from build123d import *

# Parameters (mm, degrees)
BOSS_EXTRU_2_DEPTH       = 73
ESQUISSE7_R              = 1.75
ENL_V_MAT_EXTRU_4_DEPTH  = 12
ENL_V_START              = -5.6
ENL_V_MAT_EXTRU_5_DEPTH  = 2.6
ENL_V_START_2            = -12
ESQUISSE12_R             = 1.75
ENL_V_MAT_EXTRU_6_DEPTH  = 12
ENL_V_START_3            = -3
ENL_V_MAT_EXTRU_7_DEPTH  = 2.6
ESQUISSE21_W             = 15
ESQUISSE21_H             = 17
ENL_V_MAT_EXTRU_14_DEPTH = 79.208055851
ESQUISSE22_W             = 2
ESQUISSE22_H             = 6
ENL_V_MAT_EXTRU_15_DEPTH = 79.208055851
ENL_V_START_4            = -17
ENL_V_MAT_EXTRU_17_DEPTH = 6
ENL_V_START_5            = -23
ENL_V_MAT_EXTRU_19_DEPTH = 6
CHANFREIN1_SIZE          = 4
CHANFREIN2_SIZE          = 4


with BuildPart() as part:
    # Esquisse3 → Boss.-Extru.2 (new body)
    with BuildSketch(Plane.XY):
        with BuildLine():
            ThreePointArc((-26.024027359, 27), (0, 37.5), (26.024027359, 27))
            Line((26.024027359, 27), (13.076696831, 27))
            Line((13.076696831, 27), (-13.076696831, 27))
            Line((-13.076696831, 27), (-26.024027359, 27))
        make_face()
    extrude(amount=BOSS_EXTRU_2_DEPTH)

    # Esquisse7 → Enlèv. mat.-Extru.4 (cut)
    with BuildSketch(Plane.XY.offset(73)):
        with Locations((-12.915565842, 31.180934222)):
            Circle(ESQUISSE7_R)
        with Locations((12.915565842, 31.180934222)):
            Circle(ESQUISSE7_R)
    extrude(amount=-ENL_V_MAT_EXTRU_4_DEPTH, mode=Mode.SUBTRACT)

    # Esquisse11 → Enlèv. mat.-Extru.5 (cut)
    with BuildSketch(Plane.XY.offset(73).offset(ENL_V_START)):
        with BuildLine():
            Line((-15.765565842, 31.180934222), (-15.765565842, 34.024945756))
            ThreePointArc((-15.765565842, 34.024945756), (-12.95813326, 35.190009696), (-10.065565842, 36.123875543))
            Line((-10.065565842, 36.123875543), (-10.065565842, 29.426382489))
            Line((-10.065565842, 29.426382489), (-12.915565842, 27.780934222))
            Line((-12.915565842, 27.780934222), (-15.765565842, 29.426382489))
            Line((-15.765565842, 29.426382489), (-15.765565842, 31.180934222))
        make_face()
        with BuildLine():
            Line((10.065565842, 36.123875543), (10.065565842, 29.426382489))
            Line((10.065565842, 29.426382489), (12.915565842, 27.780934222))
            Line((12.915565842, 27.780934222), (15.765565842, 29.426382489))
            Line((15.765565842, 29.426382489), (15.765565842, 34.024945756))
            ThreePointArc((15.765565842, 34.024945756), (12.95813326, 35.190009696), (10.065565842, 36.123875543))
        make_face()
    extrude(amount=ENL_V_MAT_EXTRU_5_DEPTH, mode=Mode.SUBTRACT)

    # Esquisse12 → Enlèv. mat.-Extru.6 (cut)
    with BuildSketch(Plane(origin=(0, 0, 0), x_dir=(-1, 0, 0), z_dir=(0, 0, -1)).offset(ENL_V_START_2)):
        with Locations(Location((-12.915565842, 31.180934222, 0), (0, 0, 180))):
            Circle(ESQUISSE12_R)
        with Locations(Location((12.915565842, 31.180934222, 0), (0, 0, 180))):
            Circle(ESQUISSE12_R)
    extrude(amount=ENL_V_MAT_EXTRU_6_DEPTH, mode=Mode.SUBTRACT)

    # Esquisse14 → Enlèv. mat.-Extru.7 (cut)
    with BuildSketch(Plane(origin=(0, 0, 0), x_dir=(-1, 0, 0), z_dir=(0, 0, -1)).offset(ENL_V_START_3)):
        with BuildLine():
            Line((-15.765565842, 31.689067965), (-15.765565842, 34.024945756))
            ThreePointArc((-15.765565842, 34.024945756), (-12.95813326, 35.190009696), (-10.065565842, 36.123875543))
            Line((-10.065565842, 36.123875543), (-10.065565842, 29.426382489))
            Line((-10.065565842, 29.426382489), (-12.915565842, 27.780934222))
            Line((-12.915565842, 27.780934222), (-15.765565842, 29.426382489))
            Line((-15.765565842, 29.426382489), (-15.765565842, 31.689067965))
        make_face()
        with BuildLine():
            Line((10.065565842, 36.123875543), (10.065565842, 29.426382489))
            Line((10.065565842, 29.426382489), (12.915565842, 27.780934222))
            Line((12.915565842, 27.780934222), (15.765565842, 29.426382489))
            Line((15.765565842, 29.426382489), (15.765565842, 34.024945756))
            ThreePointArc((15.765565842, 34.024945756), (12.95813326, 35.190009696), (10.065565842, 36.123875543))
        make_face()
    extrude(amount=-ENL_V_MAT_EXTRU_7_DEPTH, mode=Mode.SUBTRACT)

    # Esquisse21 → Enlèv. mat.-Extru.14 (cut, through all)
    with BuildSketch(Plane.XZ.offset(-27)):
        with Locations((0, 64.5)):
            Rectangle(ESQUISSE21_W, ESQUISSE21_H)
        with Locations((0, 8.5)):
            Rectangle(ESQUISSE21_W, ESQUISSE21_H)
    extrude(amount=-ENL_V_MAT_EXTRU_14_DEPTH, mode=Mode.SUBTRACT)

    # Esquisse22 → Enlèv. mat.-Extru.15 (cut, through all)
    with BuildSketch(Plane.XZ.offset(-27)):
        with Locations((-20, 53)):
            Rectangle(ESQUISSE22_W, ESQUISSE22_H)
        with Locations((20, 53)):
            Rectangle(ESQUISSE22_W, ESQUISSE22_H)
        with Locations((-20, 20)):
            Rectangle(ESQUISSE22_W, ESQUISSE22_H)
        with Locations((20, 20)):
            Rectangle(ESQUISSE22_W, ESQUISSE22_H)
    extrude(amount=-ENL_V_MAT_EXTRU_15_DEPTH, mode=Mode.SUBTRACT)

    # Esquisse23 → Enlèv. mat.-Extru.17 (cut)
    with BuildSketch(Plane(origin=(0, 0, 0), x_dir=(-1, 0, 0), z_dir=(0, 0, -1)).offset(ENL_V_START_4)):
        with BuildLine():
            Line((-19, 29.987497395), (-19, 32.330326321))
            ThreePointArc((-19, 32.330326321), (0, 37.5), (19, 32.330326321))
            Line((19, 32.330326321), (19, 29.987497395))
            ThreePointArc((19, 29.987497395), (0, 35.5), (-19, 29.987497395))
        make_face()
    extrude(amount=-ENL_V_MAT_EXTRU_17_DEPTH, mode=Mode.SUBTRACT)

    # Esquisse27 → Enlèv. mat.-Extru.19 (cut)
    with BuildSketch(Plane.XY.offset(73).offset(ENL_V_START_5)):
        with BuildLine():
            Line((-19, 32.330326321), (-19, 29.987497395))
            ThreePointArc((-19, 29.987497395), (0, 35.5), (19, 29.987497395))
            Line((19, 29.987497395), (19, 32.330326321))
            ThreePointArc((19, 32.330326321), (0, 37.5), (-19, 32.330326321))
        make_face()
    extrude(amount=ENL_V_MAT_EXTRU_19_DEPTH, mode=Mode.SUBTRACT)

    # Chanfrein1
    # the kernel refuses this chamfer: 4, 2.005021286 mm, written as the material it takes off along each edge
    with BuildSketch(Plane(origin=(21, 31.068472766, 56), x_dir=(0.8131904360311143, -0.581997693077495, 0), z_dir=(0, 0, -1)), Plane(origin=(21, 31.068472766, 23), x_dir=(0.8131904360311155, -0.5819976930774934, 0), z_dir=(0, 0, -1))) as chanfrein1_piece_1:
        with BuildLine():
            Line((2.009560641, 0), (CHANFREIN1_SIZE * 0.581997693077, CHANFREIN1_SIZE * 0.813190436031))
            Line((CHANFREIN1_SIZE * 0.581997693077, CHANFREIN1_SIZE * 0.813190436031), (0, 0))
            ThreePointArc((0, 0), (0.996999681, -0.013462723), (2.009560641, 0))
        make_face()
    extrude(amount=6, mode=Mode.SUBTRACT)

    # Chanfrein2
    # the kernel refuses this chamfer: 4, 2.005021286 mm, written as the material it takes off along each edge
    with BuildSketch(Plane(origin=(-21, 31.068472766, 23), x_dir=(-0.8131904360311136, -0.5819976930774963, 0), z_dir=(0, 0, -1)), Plane(origin=(-21, 31.068472766, 56), x_dir=(-0.8131904360311129, -0.581997693077497, 0), z_dir=(0, 0, -1))) as chanfrein2_piece_1:
        with BuildLine():
            Line((2.009560641, 0), (CHANFREIN2_SIZE * 0.581997693077, -CHANFREIN2_SIZE * 0.813190436031))
            Line((CHANFREIN2_SIZE * 0.581997693077, -CHANFREIN2_SIZE * 0.813190436031), (0, 0))
            ThreePointArc((0, 0), (0.996999681, 0.013462723), (2.009560641, 0))
        make_face()
    extrude(amount=6, mode=Mode.SUBTRACT)


solid = part.part
Geometry: final body of the model. Coordinates: model frame, mm. A direction names the side the tool comes from. Give positions to 0.01 mm unless a question says otherwise; leave off trailing zeros. Write each loop counter-clockwise with the first axis right and the second up, starting at its lowest first coordinate (ties: lowest second). Pieces come first, ordered by that corner, then holes.
(1) First-contact query: P1, Ø2, axis at y = 31, z = 69, coming from the -X side; P2, Ø5, axis at y = 29, z = 13.5, coming from the +X side; P3, Ø0.8, axis at y = 32.5, z = 4, coming from the +X side; P4, Ø10, axis at x = -19.5, z = 53.5, coming from the +Y side. Flat tips, straight axial feed; report the tip coordinate or a pass-through.
(2) Cut plane B-B, the plane z = 57. Return loops of the section in (x, y).
(3) Mould query, pull axis Y, two halves, no side actions, for faces 1 (the cylindrical face through (-12.108, 29.628, 64.245)), 2 (the cylindrical face through (12.54, 32.89, 1.52)), 3 (the flat face through (12, 33, 67.4)), 4 (the flat face through (14.32, 28.59, 4.28)). Classes: released by +Y, released by -Y, zero draft, split by the parting line, or undercut.
(4) Cut plane C-C, the plane x = 0.5. Return loops of the section in (y, z).
(5) Cut plane A-A, the plane z = 22. Return loops of the section in (x, y).
(6) Access query for faces 5 (the flat face through (7.5, 32, 64)), 6 (the flat face through (16, 32, 56)), 7 (the cylindrical face through (-12.108, 32.733, 1.521)). Directions: +Z, -Z, +X, -X, +Y, -Y. A direction counts if a zero-diameter tool reaches every point of the face in a straight line with its end or side. Return the directions, or none.
(7) Ray query, line 1 (Z direction, x = -13, y = 34.25); line 2 (Z direction, x = 17, y = 31.25); line 3 (Z direction, x = 6.5, y = 30.5). Return the intervals inside material, ascending.
Values follow:
1. P1: stops at x = -22.5
1. P2: stops at x = 26.02
1. P3: stops at x = 19.39
1. P4: stops at y = 34.29
2. outline: (-26.02, 27) - (-7.5, 27) - (-7.5, 36.74) arc R37.5 ccw to start; (7.5, 27) - (26.02, 27) arc R37.5 ccw to (7.5, 36.74) - close
3. face 1: undercut
3. face 2: undercut
3. face 3: zero draft
3. face 4: released by +Y
4. outline: (27, 17) - (35.5, 17) - (35.5, 23) - (37.5, 23) - (37.5, 50) - (35.5, 50) - (35.5, 56) - (27, 56) - close
5. outline: (-26.02, 27) - (-21, 27) - (-21, 27.07) - (-22.63, 29.9) arc R37.5 ccw to start; (-19, 27) - (19, 27) - (19, 29.99) arc R35.5 ccw to (-19, 29.99) - close; (21, 27) - (26.02, 27) arc R37.5 ccw to (22.63, 29.9) - (21, 27.07) - close
6. face 5: +Z, +Y, -Y
6. face 6: +Y
6. face 7: -Z
7. line 1: z = 0 to 3, 5.6 to 17, 23 to 50, 56 to 67.4, 70 to 73
7. line 2: z = 0 to 17, 23 to 50, 56 to 73
7. line 3: z = 17 to 56
